from build123d import *

# Parameters (mm, degrees)
EXTRUDE_THIN2_DEPTH = 19
BOSS_EXTRUDE1_DEPTH = 19
BOSS_EXTRUDE2_DEPTH = 1
BOSS_EXTRUDE4_DEPTH = 18


# Read off the part's stored shape, not the designer's step: Extrude-Thin2
with BuildPart() as part:
    # Extrude-Thin2 outline → Extrude-Thin2 (new body)
    with BuildSketch(Plane.XY):
        Polygon((-74.68025732, 32.45), (-73.900834456, 32), (-74.800834456, 32), (-74.800834456, -32), (-73.900834456, -32), (-74.68025732, -32.45), (-65.182845391, -48.9), (65.182845392, -48.9), (74.68025732, -32.45), (73.900834456, -32), (74.800834456, -32), (74.800834456, 32), (73.900834456, 32), (74.68025732, 32.45), (65.182845392, 48.9), (-65.182845392, 48.9), align=None)
        Polygon((-37.989647713, -32), (-46.707636777, -47.1), (-64.143614907, -47.1), (-72.861603972, -32), (-64.143614907, -16.9), (-46.707636777, -16.9), align=None, mode=Mode.SUBTRACT)
        Polygon((-36.430801986, -32.9), (-18.994823856, -32.9), (-10.796450034, -47.1), (-44.629175808, -47.1), align=None, mode=Mode.SUBTRACT)
        Polygon((-73.000834456, -3.358845727), (-65.702460634, -16), (-73.000834456, -28.641154273), align=None, mode=Mode.SUBTRACT)
        Polygon((-10.276834792, -16), (-18.994823856, -31.1), (-36.430801986, -31.1), (-45.148791051, -16), (-36.430801986, -0.9), (-18.994823856, -0.9), align=None, mode=Mode.SUBTRACT)
        Polygon((10.796450034, -47.1), (18.994823856, -32.9), (36.430801986, -32.9), (44.629175808, -47.1), align=None, mode=Mode.SUBTRACT)
        Polygon((-8.717989065, -16.9), (8.717989065, -16.9), (17.43597813, -32), (8.717989065, -47.1), (-8.717989065, -47.1), (-17.435978129, -32), align=None, mode=Mode.SUBTRACT)
        Polygon((46.707636777, -16.9), (64.143614907, -16.9), (72.861603972, -32), (64.143614907, -47.1), (46.707636777, -47.1), (37.989647713, -32), align=None, mode=Mode.SUBTRACT)
        Polygon((36.430801986, -0.9), (45.148791051, -16), (36.430801986, -31.1), (18.994823856, -31.1), (10.276834792, -16), (18.994823856, -0.9), align=None, mode=Mode.SUBTRACT)
        Polygon((73.000834456, -28.641154273), (65.702460634, -16), (73.000834456, -3.358845727), align=None, mode=Mode.SUBTRACT)
        Polygon((-37.989647713, 0), (-46.707636777, -15.1), (-64.143614907, -15.1), (-72.861603972, 0), (-64.143614907, 15.1), (-46.707636777, 15.1), align=None, mode=Mode.SUBTRACT)
        Polygon((-65.702460634, 16), (-73.000834456, 3.358845727), (-73.000834456, 28.641154273), align=None, mode=Mode.SUBTRACT)
        Polygon((-10.276834792, 16), (-18.994823856, 0.9), (-36.430801986, 0.9), (-45.148791051, 16), (-36.430801986, 31.1), (-18.994823856, 31.1), align=None, mode=Mode.SUBTRACT)
        Polygon((-37.989647713, 32), (-46.707636777, 16.9), (-64.143614907, 16.9), (-72.861603972, 32), (-64.143614907, 47.1), (-46.707636777, 47.1), align=None, mode=Mode.SUBTRACT)
        Polygon((-10.796450034, 47.1), (-18.994823856, 32.9), (-36.430801986, 32.9), (-44.629175808, 47.1), align=None, mode=Mode.SUBTRACT)
        Polygon((17.43597813, 0), (8.717989065, -15.1), (-8.717989065, -15.1), (-17.43597813, 0), (-8.717989065, 15.1), (8.717989065, 15.1), align=None, mode=Mode.SUBTRACT)
        Polygon((36.430801986, 0.9), (18.994823856, 0.9), (10.276834792, 16), (18.994823856, 31.1), (36.430801986, 31.1), (45.148791051, 16), align=None, mode=Mode.SUBTRACT)
        Polygon((72.861603972, 0), (64.143614907, -15.1), (46.707636777, -15.1), (37.989647713, 0), (46.707636777, 15.1), (64.143614907, 15.1), align=None, mode=Mode.SUBTRACT)
        Polygon((73.000834456, 28.641154273), (73.000834456, 3.358845727), (65.702460634, 16), align=None, mode=Mode.SUBTRACT)
        Polygon((17.43597813, 32), (8.717989065, 16.9), (-8.717989065, 16.9), (-17.43597813, 32), (-8.717989065, 47.1), (8.717989065, 47.1), align=None, mode=Mode.SUBTRACT)
        Polygon((36.430801986, 32.9), (18.994823856, 32.9), (10.796450034, 47.1), (44.629175808, 47.1), align=None, mode=Mode.SUBTRACT)
        Polygon((72.861603972, 32), (64.143614907, 16.9), (46.707636777, 16.9), (37.989647713, 32), (46.707636777, 47.1), (64.143614907, 47.1), align=None, mode=Mode.SUBTRACT)
    extrude(amount=EXTRUDE_THIN2_DEPTH)

    # Sketch2 → Boss-Extrude1 (add)
    with BuildSketch(Plane.XY.offset(19)):
        Polygon((73.900834456, -32), (74.68025732, -32.45), (74.800834456, -32), align=None)
        Polygon((74.68025732, 32.45), (74.800834456, 32), (73.900834456, 32), align=None)
        Polygon((-74.68025732, 32.45), (-74.800834456, 32), (-73.900834456, 32), align=None)
        Polygon((-74.68025732, -32.45), (-73.900834456, -32), (-74.800834456, -32), align=None)
    extrude(amount=-BOSS_EXTRUDE1_DEPTH)

    # Sketch3 → Boss-Extrude2 (add)
    with BuildSketch(Plane(origin=(0, 0, 0), x_dir=(-1, 0, 0), z_dir=(0, 0, -1))):
        Polygon((-74.68025732, 32.45), (-74.800834456, 32), (-74.800834456, -32), (-74.68025732, -32.45), (-65.182845392, -48.9), (65.182845391, -48.9), (74.68025732, -32.45), (74.800834456, -32), (74.800834456, 32), (74.68025732, 32.45), (65.182845392, 48.9), (-65.182845392, 48.9), align=None)
    extrude(amount=-BOSS_EXTRUDE2_DEPTH)

    # Sketch5 → Boss-Extrude4 (add)
    with BuildSketch(Plane.XY.offset(1)):
        Polygon((-73.000834456, 28.641154273), (-73.000834456, 3.358845727), (-65.702460634, 16), align=None)
        Polygon((-73.000834456, -28.641154273), (-65.702460634, -16), (-73.000834456, -3.358845727), align=None)
        Polygon((65.702460634, 16), (73.000834456, 3.358845727), (73.000834456, 28.641154273), align=None)
        Polygon((73.000834456, -3.358845727), (65.702460634, -16), (73.000834456, -28.641154273), align=None)
    extrude(amount=BOSS_EXTRUDE4_DEPTH)


solid = part.part
Build history of the part. All positions in model axes, mm. Give positions to 0.01 mm unless a question says otherwise; leave off trailing zeros. Write each loop counter-clockwise with the first axis right and the second up, starting at its lowest first coordinate (ties: lowest second). Pieces come first, ordered by that corner, then holes. Notation, with made-up numbers: (13.5, -28) - (36.5, -28) arc R19 ccw to (36.5, -16) - close; hole circle Ø11 at (-26.75, 60.5). An arc over 180 degrees is marked (long way). Use one line per item in the form item = value. Start each with the question number.
1. Band-saw the part on B-B on x = 30. Write the cut outline in (y, z), plus the area to 3 significant figures.
2. Band-saw the part on A-A on z = 10.5. Count the separate pieces of the cut face and the enclosed holes in it, plus the area to 3 significant figures.
3. Probe line 1 (Y direction, x = -8, z = 12); line 2 (Y direction, x = -21, z = 3); line 3 (X direction, y = 42.5, z = 13.75). List the from-to ranges inside material, lowest first. Write a range as [from, to].
4. Band-saw the part on D-D on x = -4. Write the cut outline in (y, z), plus the area to 3 significant figures.
5. Two-plate mould, pull along X, no slides. Class faces 1 (the face through (-70, -40.56, 9.37)), 2 (the face through (40.47, -39.9, 9.87)): released by +X, released by -X, zero draft, split by the parting line, or undercut.
6. Band-saw the part on C-C on y = 22.5. Write the cut outline in (x, z).
7. Drop flat-ended pins along their axis: pin 1 Ø1 at (x, y) = (22.5, -5.5) entering from +Z; pin 2 Ø24 at (x, y) = (7, 30) entering from +Z. Give the stop position or say it passes through.
Conclusion:
q1.outline = (-48.9, 0) - (48.9, 0) - (48.9, 19) - (47.1, 19) - (47.1, 1) - (32.9, 1) - (32.9, 19) - (31.1, 19) - (31.1, 1) - (0.9, 1) - (0.9, 19) - (-0.9, 19) - (-0.9, 1) - (-31.1, 1) - (-31.1, 19) - (-32.9, 19) - (-32.9, 1) - (-47.1, 1) - (-47.1, 19) - (-48.9, 19) - close
q1.area = 260 mm²
q2.separate_pieces = 1
q2.enclosed_holes = 17
q2.area = 2,590 mm²
q3.line_1 = [-48.9, -47.1], [-16.9, -15.1], [15.1, 16.9], [47.1, 48.9]
q3.line_2 = [-48.9, -47.1], [-32.9, -31.1], [-0.9, 0.9], [31.1, 32.9], [47.1, 48.9]
q3.line_3 = [-68.88, -66.8], [-44.05, -41.97], [-13.45, -11.37], [11.37, 13.45], [41.97, 44.05], [66.8, 68.88]
q4.outline = (-48.9, 0) - (48.9, 0) - (48.9, 19) - (47.1, 19) - (47.1, 1) - (16.9, 1) - (16.9, 19) - (15.1, 19) - (15.1, 1) - (-15.1, 1) - (-15.1, 19) - (-16.9, 19) - (-16.9, 1) - (-47.1, 1) - (-47.1, 19) - (-48.9, 19) - close
q4.area = 227 mm²
q5.face_1 = released by -X
q5.face_2 = undercut
q6.outline = (-74.8, 0) - (74.8, 0) - (74.8, 19) - (67.38, 19) - (67.38, 1) - (43.47, 1) - (43.47, 19) - (41.4, 19) - (41.4, 1) - (14.03, 1) - (14.03, 19) - (11.95, 19) - (11.95, 1) - (-11.95, 1) - (-11.95, 19) - (-14.03, 19) - (-14.03, 1) - (-41.4, 1) - (-41.4, 19) - (-43.47, 19) - (-43.47, 1) - (-67.38, 1) - (-67.38, 19) - (-74.8, 19) - close
q7.pin_1 = 1
q7.pin_2 = 19
